```python
from build123d import *

# Parameters (mm, degrees)
CUT_EXTRUDE_2_DEPTH      = 69.387157144
SKETCH_3_R               = 6
SKETCH_3_R_2             = 4
CUT_EXTRUDE_3_DEPTH      = 6
SKETCH_7_R               = 4
CUT_EXTRUDE_5_DEPTH      = 69.387157144
PATTERN_CIRCULAR_2_COUNT = 5
SKETCH_8_R               = 9.5
CUT_EXTRUDE_6_DEPTH      = 69.387157144
CUT_EXTRUDE_7_DEPTH      = 69.387157144
PATTERN_CIRCULAR_4_COUNT = 5
SKETCH_10_R              = 3
CUT_EXTRUDE_10_DEPTH     = 79.346077675
PATTERN_CIRCULAR_5_COUNT = 5


with BuildPart() as part:
    # 草图1 → 旋转1 (revolve)
    with BuildSketch(Plane.XY, mode=Mode.PRIVATE) as revolve_1_sk:
        with BuildLine():
            Line((0, 0), (-45, 0))
            Line((-45, 0), (-45, 11.036038988))
            Line((-45, 11.036038988), (-45, 32.036038988))
            ThreePointArc((-45, 32.036038988), (-42.738612788, 36.219339121), (-38, 36.618614683))
            Line((-38, 36.618614683), (-32, 34))
            Line((-32, 34), (-32, 12))
            Line((-32, 12), (0, 12))
            Line((0, 12), (0, 0))
        make_face()
    revolve(revolve_1_sk.sketch.rotate(Axis((0, 12, 0), (0, -1, 0)), 270), axis=Axis((0, 12, 0), (0, -1, 0)))

    # 草图2 → 切除-拉伸2 (cut, through all)
    with BuildSketch(Plane(origin=(0, 12, 0), x_dir=(1, 0, 0), z_dir=(0, 1, 0))):
        with BuildLine():
            ThreePointArc((-23.329642683, 21.9026887), (-30.433808521, 9.88854382), (-31.748154807, -4.00682747))
            Line((-31.748154807, -4.00682747), (-13.884121066, 1.797548946))
            ThreePointArc((-13.884121066, 1.797548946), (-13.314791228, 4.326237921), (-12.289062655, 6.706633958))
            Line((-12.289062655, 6.706633958), (-23.329642683, 21.9026887))
        make_face()
        with BuildLine():
            ThreePointArc((13.621438751, 28.956111727), (0, 32), (-13.621438751, 28.956111727))
            Line((-13.621438751, 28.956111727), (-2.580858723, 13.760056986))
            ThreePointArc((-2.580858723, 13.760056986), (0, 14), (2.580858723, 13.760056986))
            Line((2.580858723, 13.760056986), (13.621438751, 28.956111727))
        make_face()
        with BuildLine():
            Line((13.884121066, 1.797548946), (31.748154807, -4.00682747))
            ThreePointArc((31.748154807, -4.00682747), (31.93697664, -2.007367205), (32, 0))
            ThreePointArc((32, 0), (29.753559164, 11.778188191), (23.329642683, 21.9026887))
            Line((23.329642683, 21.9026887), (12.289062655, 6.706633958))
            ThreePointArc((12.289062655, 6.706633958), (13.314791228, 4.326237921), (13.884121066, 1.797548946))
        make_face()
        with BuildLine():
            ThreePointArc((10.175917134, -9.615129249), (8.228993532, -11.326237921), (6, -12.649110641))
            Line((6, -12.649110641), (6, -31.432467291))
            ThreePointArc((6, -31.432467291), (18.809128073, -25.88854382), (28.039950874, -15.419505666))
            Line((28.039950874, -15.419505666), (10.175917134, -9.615129249))
        make_face()
        with BuildLine():
            ThreePointArc((-28.039950874, -15.419505666), (-18.809128073, -25.88854382), (-6, -31.432467291))
            Line((-6, -31.432467291), (-6, -12.649110641))
            ThreePointArc((-6, -12.649110641), (-8.228993532, -11.326237921), (-10.175917134, -9.615129249))
            Line((-10.175917134, -9.615129249), (-28.039950874, -15.419505666))
        make_face()
        with BuildLine():
            ThreePointArc((28.039950874, -15.419505666), (18.809128073, -25.88854382), (6, -31.432467291))
            Line((6, -31.432467291), (6, -44.598206242))
            ThreePointArc((6, -44.598206242), (26.450336353, -36.405764747), (40.561312695, -19.487942745))
            Line((40.561312695, -19.487942745), (28.039950874, -15.419505666))
        make_face()
        with BuildLine():
            ThreePointArc((32, 0), (31.93697664, -2.007367205), (31.748154807, -4.00682747))
            Line((31.748154807, -4.00682747), (44.269516628, -8.07526455))
            ThreePointArc((44.269516628, -8.07526455), (42.797543233, 13.905764747), (31.068269874, 32.553995255))
            Line((31.068269874, 32.553995255), (23.329642683, 21.9026887))
            ThreePointArc((23.329642683, 21.9026887), (29.753559164, 11.778188191), (32, 0))
        make_face()
        with BuildLine():
            Line((-21.360065941, 39.607418282), (-13.621438751, 28.956111727))
            ThreePointArc((-13.621438751, 28.956111727), (0, 32), (13.621438751, 28.956111727))
            Line((13.621438751, 28.956111727), (21.360065941, 39.607418282))
            ThreePointArc((21.360065941, 39.607418282), (0, 45), (-21.360065941, 39.607418282))
        make_face()
        with BuildLine():
            Line((-44.269516628, -8.07526455), (-31.748154807, -4.00682747))
            ThreePointArc((-31.748154807, -4.00682747), (-30.433808521, 9.88854382), (-23.329642683, 21.9026887))
            Line((-23.329642683, 21.9026887), (-31.068269874, 32.553995255))
            ThreePointArc((-31.068269874, 32.553995255), (-42.797543233, 13.905764747), (-44.269516628, -8.07526455))
        make_face()
        with BuildLine():
            Line((-6, -44.598206242), (-6, -31.432467291))
            ThreePointArc((-6, -31.432467291), (-18.809128073, -25.88854382), (-28.039950874, -15.419505666))
            Line((-28.039950874, -15.419505666), (-40.561312695, -19.487942745))
            ThreePointArc((-40.561312695, -19.487942745), (-26.450336353, -36.405764747), (-6, -44.598206242))
        make_face()
    extrude(amount=CUT_EXTRUDE_2_DEPTH, mode=Mode.SUBTRACT)

    # 草图3 → 切除-拉伸3 (cut)
    with BuildSketch(Plane(origin=(0, 12, 0), x_dir=(1, 0, 0), z_dir=(0, 1, 0))):
        with Locations(Location((0, 32, 0), (0, 0, 270))):
            Circle(SKETCH_3_R)
        with Locations(Location((0, 32, 0), (0, 0, 270))):
            Circle(SKETCH_3_R_2, mode=Mode.SUBTRACT)
    cut_extrude_3 = extrude(amount=-CUT_EXTRUDE_3_DEPTH, mode=Mode.SUBTRACT)

    # 草图7 → 切除-拉伸5 (cut, through all)
    with BuildSketch(Plane(origin=(0, 12, 0), x_dir=(1, 0, 0), z_dir=(0, 1, 0))):
        with Locations(Location((0, 32, 0), (0, 0, 270))):
            Circle(SKETCH_7_R)
    cut_extrude_5 = extrude(amount=-CUT_EXTRUDE_5_DEPTH, mode=Mode.SUBTRACT)

    # 阵列(圆周)2: 切除-拉伸3, 切除-拉伸5 ×5 about axis
    pattern_circular_2_axis = Axis((0, 0, 0), (0, 1, 0))
    add([cut_extrude_3.rotate(pattern_circular_2_axis, i * 360 / PATTERN_CIRCULAR_2_COUNT) for i in range(1, PATTERN_CIRCULAR_2_COUNT)], mode=Mode.SUBTRACT)
    add([cut_extrude_5.rotate(pattern_circular_2_axis, i * 360 / PATTERN_CIRCULAR_2_COUNT) for i in range(1, PATTERN_CIRCULAR_2_COUNT)], mode=Mode.SUBTRACT)

    # 草图8 → 切除-拉伸6 (cut, through all)
    with BuildSketch(Plane(origin=(0, 12, 0), x_dir=(1, 0, 0), z_dir=(0, 1, 0))):
        with Locations(Location((0, 0, 0), (0, 0, 270))):
            Circle(SKETCH_8_R)
    extrude(amount=-CUT_EXTRUDE_6_DEPTH, mode=Mode.SUBTRACT)

    # 草图9 → 切除-拉伸7 (cut, through all)
    with BuildSketch(Plane(origin=(0, 12, 0), x_dir=(1, 0, 0), z_dir=(0, 1, 0))):
        with BuildLine():
            Line((-6, -12.649110641), (-6, -31.432467291))
            ThreePointArc((-6, -31.432467291), (0, -32), (6, -31.432467291))
            Line((6, -31.432467291), (6, -12.649110641))
            ThreePointArc((6, -12.649110641), (0, -14), (-6, -12.649110641))
        make_face()
    cut_extrude_7 = extrude(amount=-CUT_EXTRUDE_7_DEPTH, mode=Mode.SUBTRACT)

    # 阵列(圆周)4: 切除-拉伸7 ×5 about axis
    pattern_circular_4_axis = Axis((0, 0, 0), (0, 1, 0))
    for i in range(1, PATTERN_CIRCULAR_4_COUNT):
        add(cut_extrude_7.rotate(pattern_circular_4_axis, i * 360 / PATTERN_CIRCULAR_4_COUNT), mode=Mode.SUBTRACT)

    # 草图10 → 切除-拉伸10 (cut, through all)
    with BuildSketch(Plane(origin=(1.854101966, 0, 5.706339098), x_dir=(0.9510565162951544, 0, -0.30901699437494484), z_dir=(0.30901699437494484, 0, 0.9510565162951544))):
        with Locations((-38, 32)):
            Circle(SKETCH_10_R)
        with Locations((-38, 20)):
            Circle(SKETCH_10_R)
    cut_extrude_10 = extrude(amount=-CUT_EXTRUDE_10_DEPTH, mode=Mode.SUBTRACT)

    # 阵列(圆周)5: 切除-拉伸10 ×5 about axis
    pattern_circular_5_axis = Axis((0, 12, 0), (0, 1, 0))
    for i in range(1, PATTERN_CIRCULAR_5_COUNT):
        add(cut_extrude_10.rotate(pattern_circular_5_axis, i * 360 / PATTERN_CIRCULAR_5_COUNT), mode=Mode.SUBTRACT)


solid = part.part
```
CAD build for the part. Positions are in the model's coordinates, mm. A direction names the side the tool comes from. Round coordinates to 2 decimals unless told otherwise and drop trailing zeros. Write each loop counter-clockwise with the first axis right and the second up, starting at its lowest first coordinate (ties: lowest second). Pieces come first, ordered by that corner, then holes. Notation, with made-up numbers: (9.25, 15.25) - (40.25, 15.25) arc R32 cw to (40.25, 42.25) - close; hole circle Ø8 at (-30.5, 31.25). An arc over 180 degrees is marked (long way). Return JSON: item names as keys, results as strings. Group by question number.
Item 1: Probe probe 1 along Z at (x, y) = (12.5, 9); probe 2 along Z at (x, y) = (26, 7); probe 3 along Z at (x, y) = (-23, 21.5). List the from-to ranges inside material, lowest first.
Item 2: Band-saw the part on D-D on z = 0. List the corners of the cut face in (x, y), plus the area to 3 significant figures.
Item 3: Band-saw the part on C-C on y = 8. State how many separate pieces and enclosed holes the cut face has, plus the area to 3 significant figures.
Item 4: Flat gauge pins, fed straight in: pin 1 Ø7 at (x, z) = (-30.43, -9.89) entering from -Y; pin 2 Ø9.5 at (x, z) = (-21, 28) entering from +Y; pin 3 Ø5 at (x, z) = (17, 23) entering from +Y; pin 4 Ø8 at (y, z) = (30, 8.5) entering from -X. Where does each tip first touch, or does it go through?
Item 5: 3-axis set-ups, long thin cutter, end or side, ignore diameter. For faces 1 (the face through (0, 9, -38)), 2 (the face through (6, 24, 38)), 3 (the face through (-6, 6, 22)), 4 (the face through (17.44, 24.35, -34.21)): which of +Z, -Z, +X, -X, +Y, -Y reach the whole face in a straight line?
Item 6: Band-saw the part on B-B on z = 24. List the corners of the cut face in (x, y), plus the area to 3 significant figures.
Item 7: Mould opens along X. For faces 5 (the face through (37.921, 24.35, 6.013)), 6 (the face through (38.269, 34.028, 12.346)) say: +X half, -X half, draft (parallel to the pull), parting line (faces both ways), or undercut.
Item 8: Band-saw the part on A-A on x = 0. List the corners of the cut face in (y, z).
Resolved:
{
 "1": {"probe 1": "z = -43.23 to -27.41, -7 to 6.3, 10.37 to 43.23", "probe 2": "z = -36.73 to -13.93, -5.85 to 2.14, 14.76 to 36.73", "probe 3": "z = -38.68 to -33.47, -27.05 to -22.25"},
 "2": {"outline": "(-45, 0) - (-19.42, 0) - (-19.42, 12) - (-45, 12) - close; (-14, 0) - (-9.5, 0) - (-9.5, 12) - (-14, 12) - close; (9.5, 0) - (14, 0) - (14, 12) - (9.5, 12) - close; (19.42, 0) - (45, 0) - (45, 12) - (19.42, 12) - close", "area": "722 mm²"},
 "3": {"separate pieces": "1", "enclosed holes": "11", "area": "4,420 mm²"},
 "4": {"pin 1": "passes through", "pin 2": "stops at y = 12", "pin 3": "stops at y = 6", "pin 4": "stops at x = -44.27"},
 "5": {"face 1": "+Y", "face 2": "+Z, -Z, +X, +Y", "face 3": "+Y, -Y", "face 4": "-Z, +Y"},
 "6": {"outline": "(-38.07, 0) - (-22.34, 0) - (-22.34, 6) - (-24.5, 6) - (-24.5, 12) - (-38.07, 12) - close; (-15.28, 0) - (-6, 0) - (-6, 12) - (-13.11, 12) - (-13.11, 6) - (-15.28, 6) - close; (6, 0) - (15.28, 0) - (15.28, 6) - (13.11, 6) - (13.11, 12) - (6, 12) - close; (22.34, 0) - (38.07, 0) - (38.07, 12) - (24.5, 12) - (24.5, 6) - (22.34, 6) - close", "area": "548 mm²"},
 "7": {"face 5": "+X half", "face 6": "undercut"},
 "8": {"outline": "(0, -45) - (12, -45) - (12, -38) - (6, -38) - (6, -36) - (0, -36) - close; (0, -28) - (6, -28) - (6, -26) - (12, -26) - (12, -9.5) - (0, -9.5) - close; (0, 9.5) - (12, 9.5) - (12, 14) - (0, 14) - close; (0, 32) - (34, 32) - (36.62, 38) arc R5 ccw to (32.04, 45) - (0, 45) - close; hole circle Ø6 at (20, 38); hole circle Ø6 at (32, 38)"}
}
